from build123d import *

# Parameters (mm, degrees)
F0_W      = 488.95
F0_H      = 560.3875
F1_DEPTH  = 19.05
F3_R      = 4
F4_DEPTH  = 26.9875
F5_SIZE   = 1.5875
F13_ANGLE = 90
F22_R     = 3.175
F23_R     = 45
F24_DEPTH = 19.051


with BuildPart() as f1:
    # F0 (on Top) → F1 (new body)
    with BuildSketch(Plane.XY):
        Rectangle(F0_W, F0_H)
    extrude(amount=-F1_DEPTH)


with BuildPart() as f4:
    # F3 (on Right) → F4 (new body)
    with BuildSketch(Plane.YZ):
        with Locations((-271.8283832073, -132.3440223932)):
            Circle(F3_R)
    extrude(amount=-F4_DEPTH)

    # F5
    f5_edges = [f4.edges().sort_by_distance(p)[0] for p in [
        (-26.9875, -275.828383, -132.344022),
    ]]
    chamfer(f5_edges, length=F5_SIZE)


with BuildPart() as f6_1:
    # F6: copy of F4
    add(f4.part.moved(Location((244.475, 33.9221332073, 122.8190223932))))


with BuildPart() as f7_1:
    # F7: copy of F4
    add(f4.part.moved(Location((244.475, 129.9221332073, 122.8190223932))))


with BuildPart() as f8_1:
    # F8: copy of F4
    add(f4.part.moved(Location((244.475, 257.9221332073, 122.8190223932))))


with BuildPart() as f9_1:
    # F9: copy of F4
    add(f4.part.moved(Location((244.475, 385.9221332073, 122.8190223932))))


with BuildPart() as f10_1:
    # F10: copy of F4
    add(f4.part.moved(Location((244.475, 513.9221332073, 122.8190223932))))


with BuildPart() as f11_1:
    # F11: instance of F6_1
    add(f6_1.part.mirror(Plane.YZ))


with BuildPart() as f11_2:
    # F11: instance of F7_1
    add(f7_1.part.mirror(Plane.YZ))


with BuildPart() as f11_3:
    # F11: instance of F8_1
    add(f8_1.part.mirror(Plane.YZ))


with BuildPart() as f11_4:
    # F11: instance of F9_1
    add(f9_1.part.mirror(Plane.YZ))


with BuildPart() as f11_5:
    # F11: instance of F10_1
    add(f10_1.part.mirror(Plane.YZ))


with BuildPart() as f1_1:
    add(f1.part)

    # F12: cut F11_1, F11_2, F11_3, F11_4, F11_5, F10_1, F9_1, F8_1, F7_1, F6_1
    add(f11_1.part, mode=Mode.SUBTRACT)
    add(f11_2.part, mode=Mode.SUBTRACT)
    add(f11_3.part, mode=Mode.SUBTRACT)
    add(f11_4.part, mode=Mode.SUBTRACT)
    add(f11_5.part, mode=Mode.SUBTRACT)
    add(f10_1.part, mode=Mode.SUBTRACT)
    add(f9_1.part, mode=Mode.SUBTRACT)
    add(f8_1.part, mode=Mode.SUBTRACT)
    add(f7_1.part, mode=Mode.SUBTRACT)
    add(f6_1.part, mode=Mode.SUBTRACT)


with BuildPart() as f4_1:
    # F13: moved
    add(f4.part.rotate(Axis((244.475, -280.19375, -9.525), (0, 0, 1)), F13_ANGLE))


with BuildPart() as f16_1:
    # F16: copy of F4
    add(f4_1.part.moved(Location((-442.4846332073, 804.8625, 122.8190223932))))


with BuildPart() as f17_1:
    # F17: copy of F4
    add(f4_1.part.moved(Location((-314.4846332073, 804.8625, 122.8190223932))))


with BuildPart() as f18_1:
    # F18: copy of F4
    add(f4_1.part.moved(Location((-285.7346332073, 804.8625, 122.8190223932))))


with BuildPart() as f19_1:
    # F19: copy of F4
    add(f4_1.part.moved(Location((-157.7346332073, 804.8625, 122.8190223932))))


with BuildPart() as f4_2:
    # F20: moved
    add(f4_1.part.moved(Location((-29.7346332073, 804.8625, 122.8190223932))))


with BuildPart() as f1_2:
    add(f1_1.part)

    # F21: cut F16_1, F17_1, F18_1, F19_1, F4
    add(f16_1.part, mode=Mode.SUBTRACT)
    add(f17_1.part, mode=Mode.SUBTRACT)
    add(f18_1.part, mode=Mode.SUBTRACT)
    add(f19_1.part, mode=Mode.SUBTRACT)
    add(f4_2.part, mode=Mode.SUBTRACT)

    # F22
    f22_edges = [f1_2.edges().sort_by_distance(p)[0] for p in [
        (0, -280.19375, -19.05),
        (0, -280.19375, 0),
    ]]
    fillet(f22_edges, radius=F22_R)

    # F23 (on face) → F24 (cut, through all)
    with BuildSketch(Plane.XY):
        with Locations((0, 203.99375)):
            Circle(F23_R)
    extrude(amount=-F24_DEPTH, mode=Mode.SUBTRACT)


solid = f1_2.part
Check sheet for the modelled part. Datum: model origin and axes. Units: mm. Give positions to 0.01 mm unless a question says otherwise; leave off trailing zeros. Write each loop counter-clockwise with the first axis right and the second up, starting at its lowest first coordinate (ties: lowest second). Pieces come first, ordered by that corner, then holes. Notation, with made-up numbers: (-4, 88) -> (15, 88) arc R23 ccw to (15, 105) -> close; hole circle Ø4 at (67, -37.75). An arc over 180 degrees is marked (long way). One line per item, written item: value. Start each with the question number.
Item 1: Gauge pin test, flat ends, axial feed: pin 1 (6.5 mm diameter, centred on y = 114.09, z = -9.52, fed in from -X); pin 2 (1.4 mm diameter, centred on x = -48.5, z = -9, fed in from +Y); pin 3 (4 mm diameter, centred on y = -141, z = -8.5, fed in from -X). Record the tip position at first contact, or that the pin passes through.
Item 2: Section check A-A on x = 0. Record the cut outline in (y, z) (3 decimals).
Item 3: Draft check along Y on faces 1 (the flat face through (-3, 280.194, -9)), 2 (the cylindrical face through (20.76, 164.07, -9.39)), 3 (the flat face through (244.475, -4, -9)). Enter one of: +Y half, -Y half, draft (parallel to the pull), parting line (faces both ways), or undercut.
Item 4: Material ranges on probe 1 along Y at (x, z) = (-72, -16.5); probe 2 along Y at (x, z) = (-11, -17.5); probe 3 along Y at (x, z) = (-26.5, -2.5), recorded low to high. Write a range as from..to.
Results list:
1. pin 1: x = -218.33
1. pin 2: y = 253.21
1. pin 3: x = -218.44
2. outline: (-280.194, -15.875) arc R3.175 ccw to (-277.019, -19.05) -> (158.994, -19.05) -> (158.994, 0) -> (-277.019, 0) arc R3.175 ccw to (-280.194, -3.175) -> close; (248.994, -19.05) -> (280.194, -19.05) -> (280.194, 0) -> (248.994, 0) -> close
3. face 1: +Y half
3. face 2: undercut
3. face 3: draft
4. probe 1: -280.13..280.19
4. probe 2: -279.75..160.36, 247.63..280.19
4. probe 3: -280.12..167.62, 240.36..280.19
